The model under review builds one solid part; all positions refer to its coordinate system, in mm. Face numbers are marked on the shaded views. Give positions to 0.01 mm unless a question says otherwise; leave off trailing zeros. Loops run counter-clockwise (first coordinate to the right, second up) from the corner with the lowest first, then second, coordinate; pieces in that order, holes last. Notation, with made-up numbers: M 3,63.25 L 43,63.25 A22 cw 43,77.25 Z; hole C 12.5,-9.5 d9. An arc over 180 degrees is marked long. Return JSON: item names as keys, results as strings. Group by question number.
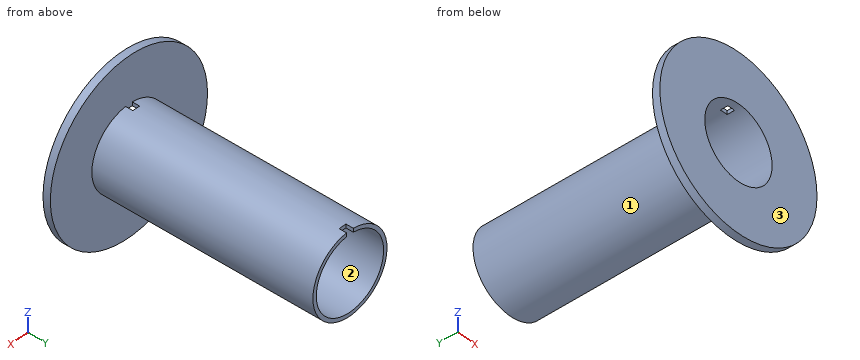
```python
from build123d import *

# Parameters (mm, degrees)
SKETCH1_R           = 88.9
SKETCH1_R_2         = 38.1
BOSS_EXTRUDE1_DEPTH = 7.62
SKETCH2_R           = 41.91
SKETCH2_R_2         = 38.1
BOSS_EXTRUDE2_DEPTH = 228.6
SKETCH3_W           = 7.62
SKETCH3_H           = 7.62
CUT_EXTRUDE1_DEPTH  = 89.9


with BuildPart() as part:
    # Sketch1 → Boss-Extrude1 (new body)
    with BuildSketch(Plane(origin=(0, 0, 0), x_dir=(1, 0, 0), z_dir=(0, 1, 0))):
        Circle(SKETCH1_R)
        Circle(SKETCH1_R_2, mode=Mode.SUBTRACT)
    extrude(amount=BOSS_EXTRUDE1_DEPTH)

    # Sketch2 → Boss-Extrude2 (add)
    with BuildSketch(Plane(origin=(0, 7.62, 0), x_dir=(1, 0, 0), z_dir=(0, 1, 0))):
        Circle(SKETCH2_R)
        Circle(SKETCH2_R_2, mode=Mode.SUBTRACT)
    extrude(amount=BOSS_EXTRUDE2_DEPTH)

    # Sketch3 → Cut-Extrude1 (cut, through all)
    with BuildSketch(Plane.XY):
        with Locations((0, 11.43)):
            Rectangle(SKETCH3_W, SKETCH3_H)
        with Locations((0, 232.41)):
            Rectangle(SKETCH3_W, SKETCH3_H)
    extrude(amount=CUT_EXTRUDE1_DEPTH, mode=Mode.SUBTRACT)


solid = part.part
```
(1) Add section C-C (x = -20.5). Write out the cut boundary in (y, z), and give its area (3 significant figures).
(2) For probe 1 along Z at (x, y) = (0, 178); probe 2 along Y at (x, z) = (-29, -47), list the stretches that pass through material, from the lowest coordinate up.
(3) Add section B-B (z = 0). Write out the cut boundary in (x, y).
(4) For pin 1 (4 mm diameter, centred on y = 12.5, z = 39.5, fed in from -X); pin 2 (1 mm diameter, centred on y = 42, z = -16.5, fed in from +X); pin 3 (12 mm diameter, centred on y = 89.5, z = -20, fed in from +X), all flat-tipped, find the tip position at first contact; note any pin that passes through.
(5) Mouldability with a two-part tool opening along X and no side actions: class the marked faces 1, 2 and 3 as released by +X, released by -X, zero draft, split by the parting line, or undercut.
(6) Add section A-A (x = 0). Write out the cut boundary in (y, z).
(7) Add section D-D (y = 206.5). Write out the cut boundary in (x, z).
Verdict:
{
 "1": {"outline": "M 0,-86.5 L 7.62,-86.5 L 7.62,-36.55 L 236.22,-36.55 L 236.22,-32.11 L 0,-32.11 Z; M 0,32.11 L 236.22,32.11 L 236.22,36.55 L 7.62,36.55 L 7.62,86.5 L 0,86.5 Z", "area": "2,860 mm²"},
 "2": {"probe 1": "z = -41.91 to -38.1, 38.1 to 41.91", "probe 2": "y = 0 to 7.62"},
 "3": {"outline": "M -88.9,0 L -38.1,0 L -38.1,236.22 L -41.91,236.22 L -41.91,7.62 L -88.9,7.62 Z; M 38.1,0 L 88.9,0 L 88.9,7.62 L 41.91,7.62 L 41.91,236.22 L 38.1,236.22 Z"},
 "4": {"pin 1": "stops at x = -18.71", "pin 2": "stops at x = 38.74", "pin 3": "stops at x = 39.5"},
 "5": {"face 1": "split by the parting line", "face 2": "undercut", "face 3": "zero draft"},
 "6": {"outline": "M 0,-88.9 L 7.62,-88.9 L 7.62,-41.91 L 236.22,-41.91 L 236.22,-38.1 L 0,-38.1 Z; M 0,38.1 L 7.62,38.1 L 7.62,88.9 L 0,88.9 Z; M 15.24,38.1 L 228.6,38.1 L 228.6,41.91 L 15.24,41.91 Z"},
 "7": {"outline": "C 0,0 d83.82; hole C 0,0 d76.2"}
}
